```python
from build123d import *

# Parameters (mm, degrees)
SKETCH_1_W      = 260
SKETCH_1_H      = 120
EXTRUDE_1_DEPTH = 35
FILLET_1_R      = 8
FILLET_2_R      = 3
SKETCH_2_R      = 3.5
EXTRUDE_2_DEPTH = 20


with BuildPart() as part:
    # 草图1 → 凸台-拉伸1 (new, symmetric)
    with BuildSketch(Plane(origin=(0, 0, 0), x_dir=(1, 0, 0), z_dir=(0, 1, 0))):
        Rectangle(SKETCH_1_W, SKETCH_1_H)
    extrude(amount=EXTRUDE_1_DEPTH, both=True)

    # 圆角1
    fillet_1_edges = [part.edges().sort_by_distance(p)[0] for p in [
        (-130, 0, -60),
        (130, 0, -60),
        (130, 0, 60),
        (-130, 0, 60),
    ]]
    fillet(fillet_1_edges, radius=FILLET_1_R)

    # 圆角2
    fillet_2_edges = [part.edges().sort_by_distance(p)[0] for p in [
        (0, -35, -60),
        (0, 35, -60),
        (-130, -35, 0),
        (130, -35, 0),
        (0, -35, 60),
        (-127.656854249, -35, -57.656854249),
        (-127.656854249, -35, 57.656854249),
        (127.656854249, -35, 57.656854249),
        (127.656854249, -35, -57.656854249),
        (130, 35, 0),
        (-130, 35, 0),
        (0, 35, 60),
        (-127.656854249, 35, -57.656854249),
        (-127.656854249, 35, 57.656854249),
        (127.656854249, 35, 57.656854249),
        (127.656854249, 35, -57.656854249),
    ]]
    fillet(fillet_2_edges, radius=FILLET_2_R)

    # 草图2 → 凸台-拉伸2 (add, symmetric)
    with BuildSketch(Plane.ZY.offset(130)):
        with Locations(Location((-56.5, 4, 0), (0, 0, 180))):
            Circle(SKETCH_2_R)
        with Locations(Location((-56.5, -4, 0), (0, 0, 180))):
            Circle(SKETCH_2_R)
    extrude(amount=EXTRUDE_2_DEPTH, both=True)


solid = part.part
```
Source: CAD feature listing. Evaluate the final solid. Frame: model axes, mm. A direction names the side the tool comes from. Give positions to 0.01 mm unless a question says otherwise; leave off trailing zeros. Loops run counter-clockwise (first coordinate to the right, second up) from the corner with the lowest first, then second, coordinate; pieces in that order, holes last. Notation, with made-up numbers: (46.5, 52) - (60.5, 52) arc R14 cw to (60.5, 58) - close; hole circle Ø10 at (5.25, 70.25). An arc over 180 degrees is marked (long way). Use CSV: the item, a comma, the result in double quotes. Start each with the question number.
1. Draft query along Y for faces 1 (the flat face through (-150, 4, -56)), 2 (the flat face through (-2, 35, -1)), 3 (the cylindrical face through (-139.31, -5.05, -59.84)). Return one class per face: +Y half, -Y half, draft (parallel to the pull), parting line (faces both ways), or undercut.
2. Section A-A (z = 5). Output: boundary loops of the cut face in (x, y), then the cut area to 3 significant figures.
3. Section B-B (y = 24.5). Output: boundary loops of the cut face in (x, z), then the cut area to 3 significant figures.
4. Ray query, L1, parallel to X at y = 25, z = 50; L2, parallel to X at y = 15.5, z = -55. Return the intervals inside material, ascending.
5. Reachability of faces 4 (the cylindrical face through (-139.31, 2.95, -59.84)), 5 (the cylindrical face through (127.719, 0.448, 57.594)) from +Z, -Z, +X, -X, +Y, -Y: full face, straight path, thin tool, end or side. Return the list, or none.
Response:
1,face 1,"draft"
1,face 2,"+Y half"
1,face 3,"undercut"
2,outline,"(-130, -32) arc R3 ccw to (-127, -35) - (127, -35) arc R3 ccw to (130, -32) - (130, 32) arc R3 ccw to (127, 35) - (-127, 35) arc R3 ccw to (-130, 32) - close"
2,area,"18,200 mm²"
3,outline,"(-130, -52) arc R8 ccw to (-122, -60) - (122, -60) arc R8 ccw to (130, -52) - (130, 52) arc R8 ccw to (122, 60) - (-122, 60) arc R8 ccw to (-130, 52) - close"
3,area,"31,100 mm²"
4,L1,"-130 to 130"
4,L2,"-129.42 to 129.42"
5,face 4,"-X"
5,face 5,"+Z, +X, +Y, -Y"
